Check sheet for the drawn part. Datum: minimum x, y, z corner. Units: mm. Round coordinates to 2 decimals unless told otherwise and drop trailing zeros. Write each loop counter-clockwise with the first axis right and the second up, starting at its lowest first coordinate (ties: lowest second). Pieces come first, ordered by that corner, then holes. Notation, with made-up numbers: (56.25, 15) - (66.25, 15) arc R24 cw to (66.25, 54) - close; hole circle Ø3 at (67.5, -1.5). An arc over 180 degrees is marked (long way). Answer as a JSON object with one key per item and string values.
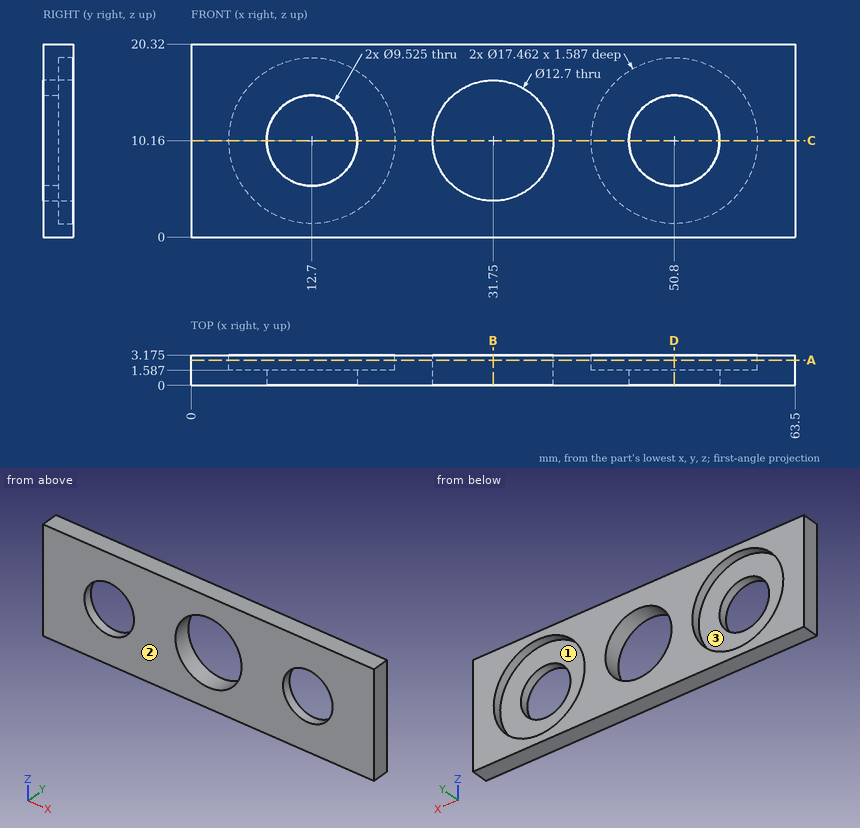
Q1. Section check C-C, the plane z = 10.16. Record the cut outline in (x, y) (1 decimal).
Geometry check:
{"outline": "(0, 0) - (7.9, 0) - (7.9, 1.6) - (4, 1.6) - (4, 3.2) - (0, 3.2) - close; (17.5, 0) - (25.4, 0) - (25.4, 3.2) - (21.4, 3.2) - (21.4, 1.6) - (17.5, 1.6) - close; (38.1, 0) - (46, 0) - (46, 1.6) - (42.1, 1.6) - (42.1, 3.2) - (38.1, 3.2) - close; (55.6, 0) - (63.5, 0) - (63.5, 3.2) - (59.5, 3.2) - (59.5, 1.6) - (55.6, 1.6) - close"}
Q2. Material ranges on line 1 along X through (y, z) = (2.1, 10.16); line 2 along X through (y, z) = (0.4, 10.16); line 3 along Z through (x, y) = (50.8, 1.15), recorded low to high. Write a range as [from, to].
Geometry check:
{"line 1": "x = [0, 3.97], [21.43, 25.4], [38.1, 42.07], [59.53, 63.5]", "line 2": "x = [0, 7.94], [17.46, 25.4], [38.1, 46.04], [55.56, 63.5]", "line 3": "z = [0, 5.4], [14.92, 20.32]"}
Q3. Section check B-B, the plane x = 31.75. Record the cut outline in (y, z) (1 decimal), then the cut area to 3 significant figures.
Geometry check:
{"outline": "(0, 0) - (3.2, 0) - (3.2, 3.8) - (0, 3.8) - close; (0, 16.5) - (3.2, 16.5) - (3.2, 20.3) - (0, 20.3) - close", "area": "24.2 mm2"}
Q4. Section check D-D, the plane x = 50.8. Record the cut outline in (y, z) (1 decimal).
Geometry check:
{"outline": "(0, 0) - (3.2, 0) - (3.2, 1.4) - (1.6, 1.4) - (1.6, 5.4) - (0, 5.4) - close; (0, 14.9) - (1.6, 14.9) - (1.6, 18.9) - (3.2, 18.9) - (3.2, 20.3) - (0, 20.3) - close"}
Q5. Gauge pin test, flat end, axial feed: P1, Ø8.5, axis at x = 49.5, z = 10.5, coming from the +Y side. Record the tip position at first contact, or that the pin passes through.
Geometry check:
{"P1": "stops at y = 1.59"}
Q6. Release check for a two-part mould opening along Z. For the marked faces 1, 2 and 3 record: released by +Z, released by -Z, zero draft, split by the parting line, or undercut.
Geometry check:
{"face 1": "undercut", "face 2": "zero draft", "face 3": "undercut"}
Q7. Section check A-A, the plane y = 2.65. Record the cut outline in (x, z).
Geometry check:
{"outline": "(0, 0) - (63.5, 0) - (63.5, 20.32) - (0, 20.32) - close; hole circle Ø17.46 at (12.7, 10.16); hole circle Ø12.7 at (31.75, 10.16); hole circle Ø17.46 at (50.8, 10.16)"}
